Read the model definition and answer for the solid it produces. Units are mm, in the model's axes. A direction names the side the tool comes from. Give positions to 0.01 mm unless a question says otherwise; leave off trailing zeros. Write each loop counter-clockwise with the first axis right and the second up, starting at its lowest first coordinate (ties: lowest second). Pieces come first, ordered by that corner, then holes. Notation, with made-up numbers: (-31, -7) -> (-16, -7) arc R18 cw to (-16, 27) -> close; hole circle Ø8 at (-40, -8.5). An arc over 180 degrees is marked (long way). Answer as CSV lines item,"result". Start each with the question number.
1. A tool of negligible diameter and unlimited length cuts with its end or side. For faces 1 (the cylindrical face through (5.294, 12.747, 0.273)), 2 (the cylindrical face through (5.7, 7.5, 5)), from which of +Z, -Z, +X, -X, +Y, -Y can it reach the whole face along a straight path? Write none if from no direction.
2. Find the intervals of material crossed by line 1 (Z direction, x = 5.5, y = 2.5); line 2 (X direction, y = 7.25, z = 9) (3 decimals); line 3 (Y direction, x = 4, z = 8), in increasing order.
3. The part is cut by section D-D, the plane x = 3.25. Determine the outline of the cut face in (y, z), and give its area (3 significant figures).
4. The part is cut by section B-B, the plane z = 0. Determine the outline of the cut face in (x, y), and give its area (3 significant figures).
5. For a pull along X with two mould halves and no side action, classify faces 3 (the flat face through (10.2, 6, 0)), 4 (the flat face through (6, 0.5, 7)), 5 (the flat face through (1.02, 7, 0)), 6 (the cylindrical face through (5.5, 7.5, -5)) as pulls with the +X half, pulls with the -X half, needs draft (parallel to the pull), parting line crosses it, or undercut.
6. Given pin 1 (1 mm diameter, centred on x = 6, y = 3.5, fed in from -Z); pin 2 (5.5 mm diameter, centred on x = 5.605, z = -9, fed in from +Y); pin 3 (5 mm diameter, centred on x = 8.5, y = 10.5, fed in from -Z), each flat-ended and moving along its own axis, determine where each tip first touches the part or whether it passes through.
7. The part is cut by section A-A, the plane x = 6. Determine the outline of the cut face in (y, z).
8. The part is cut by section C-C, the plane y = 3.5. Give the number of separate pieces and of enclosed holes in the cut face, and give its area (3 significant figures).
Autodesk Inventor part; units mm, degrees
ref_plane "part2_to_part1_XY" through (0, 0, 0) normal (1, 0, 0) x (0, 0, -1)
ref_plane "part2_to_part1_YZ" through (0, 0, 0) normal (0, 0, -1) x (0, 1, 0)
ref_plane "part2_to_part1_ZX" through (0, 0, 0) normal (0, 1, 0) x (1, 0, 0)
sketch "Sketch_1" plane through (0, 0, 0) normal (0, 0, 1) x (1, 0, 0)
  line L0 (10.2, 0) -> (0, 0)
  line L1 (1.02, 5.1) -> (10.2, 5.1)
  line L2 (10.2, 5.1) -> (10.2, 12.24)
  line L3 (10.2, 12.24) -> (9.69, 12.75)
  line L4 (9.69, 12.75) -> (1.02, 12.75)
  line L5 (1.02, 12.75) -> (1.02, 5.1)
  dimension "d15" = 5.1
revolve "Revolution1" add sketch "Sketch_1" angle 180 mid plane about axis through (10.2, 0, 0) along (-1, 0, 0)
sketch "Sketch_2" plane through (0, 0, 0) normal (0, 0, 1) x (1, 0, 0)
  line L0 (0, 0.5) -> (0, 0)
  line L1 (0, 0) -> (20, 0)
  line L2 (20, 0) -> (20, 0.5)
  line L3 (20, 0.5) -> (0, 0.5)
extrude "Extrusion1" cut sketch "Sketch_2" along normal mid plane 50
ref_plane "part2_to_part1_XY" through (0, 0, 0) normal (1, 0, 0) x (0, 0, -1)
ref_plane "part2_to_part1_YZ" through (0, 0, 0) normal (0, 0, -1) x (0, 1, 0)
ref_plane "part2_to_part1_ZX" through (0, 0, 0) normal (0, 1, 0) x (1, 0, 0)
ref_plane "part2_to_screw1_XY" through (5.5, 4.5, 9) normal (0, 1, 0) x (1, 0, 0)
ref_plane "part2_to_screw1_YZ" through (5.5, 4.5, 9) normal (1, 0, 0) x (0, 0, -1)
ref_plane "part2_to_screw1_ZX" through (5.5, 4.5, 9) normal (0, 0, -1) x (0, 1, 0)
ref_plane "part2_to_screw2_XY" through (5.5, 4.5, -9) normal (0, 1, 0) x (1, 0, 0)
ref_plane "part2_to_screw2_YZ" through (5.5, 4.5, -9) normal (1, 0, 0) x (0, 0, -1)
ref_plane "part2_to_screw2_ZX" through (5.5, 4.5, -9) normal (0, 0, -1) x (0, 1, 0)
ref_plane "作業平面10" through (5.355, 12.75, 0) normal (0, 1, 0) x (-1, 0, 0)
sketch "スケッチ6" plane through (5.355, 12.75, 0) normal (0, 1, 0) x (-1, 0, 0)
  circle A0 centre (-0.25, -9) radius 2.25
  circle A1 centre (-0.25, -9) radius 4
  circle A2 centre (-0.25, -9) radius 1.7
  circle A3 centre (-0.25, 9) radius 2.25
  circle A4 centre (-0.25, 9) radius 4
  circle A5 centre (-0.25, 9) radius 1.7
  point P0 (5.355, 0)
  dimension "d7" = 8
  dimension "d8" = 3.4
  dimension "d9" = 8
  dimension "d10" = 3.4
extrude "押し出し2" cut sketch "スケッチ6" against normal through all contours A2 | A5
extrude "押し出し3" cut sketch "スケッチ6" against normal blind 8 contours A0 | A1 | A2 | A3 | A4 | A5
properties part number "MBRDAC45-2-10_p2"
Results found:
1,face 1,"+X, -X, +Y"
1,face 2,"+Y"
2,line 1,"z = -12.5 to -10.7, -7.3 to -4.45, 4.45 to 7.3, 10.7 to 12.5"
2,line 2,"x = 1.02 to 1.605, 9.605 to 10.2"
2,line 3,"y = 0.5 to 4.75"
3,outline,"(0.5, -12.74) arc R12.75 ccw to (4.75, -11.83) -> (4.75, -5.77) -> (11.37, -5.77) arc R12.75 ccw to (11.37, 5.77) -> (4.75, 5.77) -> (4.75, 11.83) arc R12.75 ccw to (0.5, 12.74) -> (0.5, 5.08) arc R5.1 cw to (0.5, -5.08) -> close"
3,area,"157 mm²"
4,outline,"(1.02, 5.1) -> (10.2, 5.1) -> (10.2, 12.24) -> (9.69, 12.75) -> (1.02, 12.75) -> close"
4,area,"70.1 mm²"
5,face 3,"pulls with the +X half"
5,face 4,"needs draft"
5,face 5,"pulls with the -X half"
5,face 6,"undercut"
6,pin 1,"stops at z = -12.39"
6,pin 2,"stops at y = 4.75"
6,pin 3,"stops at z = -9.74"
7,outline,"(0.5, -12.74) arc R12.75 ccw to (4.75, -11.83) -> (4.75, -10.65) -> (0.5, -10.65) -> close; (0.5, -7.35) -> (4.75, -7.35) -> (4.75, -5.02) -> (11.72, -5.02) arc R12.75 ccw to (11.72, 5.02) -> (4.75, 5.02) -> (4.75, 7.35) -> (0.5, 7.35) -> (0.5, 5.08) arc R5.1 cw to (0.5, -5.08) -> close; (0.5, 10.65) -> (4.75, 10.65) -> (4.75, 11.83) arc R12.75 ccw to (0.5, 12.74) -> close"
8,separate pieces,"2"
8,enclosed holes,"2"
8,area,"139 mm²"
